Design review of the part built by this model. Coordinates are the model's own, in mm. A direction names the side the tool comes from. Round coordinates to 2 decimals unless told otherwise and drop trailing zeros. Order: outer loops, then holes, each group sorted by start corner. A loop starts at its lowest first (then second) coordinate and runs counter-clockwise, first axis right, second up. Notation, with made-up numbers: (14, -37) - (32, -37) arc R12 cw to (32, -18) - close; hole circle Ø10 at (19.25, 50). An arc over 180 degrees is marked (long way). Write item = value, one per line.
from build123d import *

# Parameters (mm, degrees)
F0_R     = 50
F0_R_2   = 7
F1_DEPTH = 5
F2_SIZE  = 0.7
F3_R     = 28
F4_DEPTH = 3
F5_DEPTH = 3


with BuildPart() as f1:
    # F0 (on Top) → F1 (new body)
    with BuildSketch(Plane.XY):
        Circle(F0_R)
        with Locations((-13.5, 10)):
            Circle(F0_R_2, mode=Mode.SUBTRACT)
        with Locations((13.5, 10)):
            Circle(F0_R_2, mode=Mode.SUBTRACT)
    extrude(amount=F1_DEPTH)

    # F2
    f2_edges = [f1.edges().sort_by_distance(p)[0] for p in [
        (-50, 0, 0),
        (50, 0, 2.5),
        (-50, 0, 5),
    ]]
    chamfer(f2_edges, length=F2_SIZE)

    # F3 (on face) → F4 (join)
    with BuildSketch(Plane.XY.offset(5)):
        Circle(F3_R)
    extrude(amount=F4_DEPTH)

    # F5 (cut, through all): faces of the model
    f5_faces = [f1.faces().sort_by_distance(p)[0] for p in [
        (-13.5, 10, 5),
        (13.5, 10, 5),
    ]]
    extrude(f5_faces, amount=-F5_DEPTH, mode=Mode.SUBTRACT)


solid = f1.part
1) Clearance check with flat-ended pins moving along their axes: pin 1 Ø1.5 at (x, z) = (12, 1.5) entering from -Y; pin 2 Ø4 at (x, z) = (3.5, 5) entering from +Y; pin 3 Ø22.5 at (x, y) = (-13.5, 10) entering from -Z; pin 4 Ø3 at (x, z) = (6.5, 5) entering from +Y. State where each tip first meets the part, or that it passes through.
Findings:
pin_1 = -48.72
pin_2 = 49.97
pin_3 = 0
pin_4 = 49.73
2) To check wall thickness, follow L1, parallel to X at y = 13, z = 1.5; L2, parallel to Z at x = 36.5, y = 32.5; L3, parallel to Y at x = -13.5, z = 3.75. State the ranges of each line that lie inside material, in increasing order. Write a range as from..to.
Findings:
L1 = -48.28..-19.82, -7.18..7.18, 19.82..48.28
L2 = 0..5
L3 = -48.14..3, 17..48.14
3) We need section D-D on y = 10. Give the number of separate pieces and of enclosed holes in the cut face, and give its area (3 significant figures).
Findings:
separate_pieces = 3
enclosed_holes = 0
area = 422 mm^2
4) For faces 1 (the cylindrical face through (25.865, -10.724, 6.479)), 2 (the flat face through (-1, 1, 0)), list the 3-axis set-ups (+Z, -Z, +X, -X, +Y, -Y) from which the entire face can be reached by the end or side of a thin tool; tool diameter is ignored.
Findings:
face_1 = +Z
face_2 = -Z, +X, -X, +Y, -Y
5) We need section C-C on z = 2.5. Write out the cut boundary in (x, y).
Findings:
outline = circle Ø100 at (0, 0); hole circle Ø14 at (-13.5, 10); hole circle Ø14 at (13.5, 10)
6) The part is to be moulded in two halves that separate along X. For faces 3 (the flat face through (0, 0, 8)), 4 (the cylindrical face through (47.69, 15.02, 2.47)), 5 (the cylindrical face through (7.945, 5.741, 3.944)), 6 (the cylindrical face through (-20.493, 10.308, 3.944)), say which applies: released by +X, released by -X, zero draft, split by the parting line, or undercut.
Findings:
face_3 = zero draft
face_4 = split by the parting line
face_5 = undercut
face_6 = undercut
7) We need section A-A on y = 0. Write out the cut boundary in (x, z).
Findings:
outline = (-50, 0.7) - (-49.3, 0) - (49.3, 0) - (50, 0.7) - (50, 4.3) - (49.3, 5) - (28, 5) - (28, 8) - (-28, 8) - (-28, 5) - (-49.3, 5) - (-50, 4.3) - close
